Can you work these out from the model? Positions are in its coordinate system, mm. A direction names the side the tool comes from. Coordinates: 2 decimals unless noted, no trailing zeros. Order: outer loops, then holes, each group sorted by start corner. A loop starts at its lowest first (then second) coordinate and runs counter-clockwise, first axis right, second up. Notation, with made-up numbers: (86.25, 23) -> (140.25, 23) arc R13 ccw to (140.25, 48) -> close; hole circle Ø10 at (73, -7.5). An arc over 180 degrees is marked (long way). Write item = value, one per line. Start each with the question number.
Autodesk Inventor part; units mm, degrees
ref_plane "YZ Plane" through (0, 0, 0) normal (1, 0, 0) x (0, 1, 0)
ref_plane "XZ Plane" through (0, 0, 0) normal (0, 1, 0) x (-1, 0, 0)
ref_plane "XY Plane" through (0, 0, 0) normal (0, 0, 1) x (1, 0, 0)
sketch "Sketch1" plane through (0, 0, 0) normal (0, 0, 1) x (1, 0, 0)
  line L0 (-60.5, -49.5) -> (60.5, -49.5)
  line L1 (60.5, -49.5) -> (60.5, 49.5)
  line L2 (60.5, 49.5) -> (-60.5, 49.5)
  line L3 (-60.5, 49.5) -> (-60.5, -49.5)
  line L4 (-60.5, -49.5) -> (60.5, 49.5) construction
  line L5 (60.5, -49.5) -> (-60.5, 49.5) construction
  point P0 (0, 0)
  dimension "d0" = 121
  dimension "d1" = 99
extrude "Extrusion1" add sketch "Sketch1" along normal blind 37
sketch "Sketch3" plane through (0, 0, 37) normal (0, 0, 1) x (1, 0, 0)
  line L0 (-58.5, -47.5) -> (58.5, -47.5)
  line L1 (58.5, -47.5) -> (58.5, 47.5)
  line L2 (58.5, 47.5) -> (-58.5, 47.5)
  line L3 (-58.5, 47.5) -> (-58.5, -47.5)
  line L4 (-58.5, -47.5) -> (58.5, 47.5) construction
  line L5 (58.5, -47.5) -> (-58.5, 47.5) construction
  point P0 (0, 0)
  dimension "d8" = 117
  dimension "d9" = 95
extrude "Extrusion3" cut sketch "Sketch3" against normal blind 35.3
sketch "Sketch4" plane through (0, 0, 1.7) normal (0, 0, 1) x (1, 0, 0)
  line L0 (5.5, -22.5) -> (8.5, -22.5)
  line L1 (8.5, -22.5) -> (8.5, 22.5)
  line L2 (8.5, 22.5) -> (5.5, 22.5)
  line L3 (5.5, 22.5) -> (5.5, -22.5)
  line L4 (5.5, -22.5) -> (8.5, 22.5) construction
  line L5 (8.5, -22.5) -> (5.5, 22.5) construction
  line L6 (-58.5, -47.5) -> (-58.5, 47.5)
  point P0 (0, 0)
  point P1 (7, 0)
  dimension "d12" = 3
  dimension "d13" = 65.5
  dimension "d14" = 45
extrude "Extrusion4" add sketch "Sketch4" along normal blind 4
sketch "Sketch5" plane through (-60.5, 49.5, 0) normal (0, -1, 0) x (1, 0, 0)
  circle A0 centre (79, 8.7) radius 3
  line L0 (119, 1.7) -> (2, 1.7)
  line L1 (69, 1.7) -> (69, 5.7)
  point P0 (60.5, 0)
  dimension "d17" = 6
  dimension "d18" = 7
  dimension "d19" = 10
extrude "Extrusion5" cut sketch "Sketch5" along normal blind 4
sketch "Sketch6" plane through (-60.5, 49.5, 0) normal (0, -1, 0) x (1, 0, 0)
  line L0 (89.25, 5.5) -> (108.75, 5.5)
  line L1 (108.75, 5.5) -> (108.75, 18.5)
  line L2 (108.75, 18.5) -> (89.25, 18.5)
  line L3 (89.25, 18.5) -> (89.25, 5.5)
  line L4 (89.25, 5.5) -> (108.75, 18.5) construction
  line L5 (108.75, 5.5) -> (89.25, 18.5) construction
  line L6 (0, 0) -> (121, 0)
  circle A0 centre (79, 8.7) radius 3
  point P0 (60.5, 0)
  point P1 (99, 12)
  point P2 (79, 9)
  dimension "d23" = 19.5
  dimension "d24" = 13
  dimension "d25" = 12
  dimension "d26" = 20
extrude "Extrusion6" cut sketch "Sketch6" along normal blind 4 contours L3 L2 L1 L0
sketch "Sketch9" plane through (60.5, -49.5, 0) normal (1, 0, 0) x (0, 0, -1)
  line L0 (-25, 43.5) -> (-29, 43.5)
  line L1 (-29, 43.5) -> (-29, 55.5)
  line L2 (-29, 55.5) -> (-25, 55.5)
  line L3 (-25, 55.5) -> (-25, 43.5)
  line L4 (-25, 43.5) -> (-29, 55.5) construction
  line L5 (-29, 43.5) -> (-25, 55.5) construction
  line L6 (-37, 0) -> (-37, 99)
  point P0 (0, 49.5)
  point P1 (-27, 49.5)
  point P2 (-27, 49.5)
  point P3 (-37, 49.5)
  dimension "d37" = 12
  dimension "d38" = 4
  dimension "d39" = 10
extrude "Extrusion8" cut sketch "Sketch9" against normal blind 10
fillet "Fillet2" radius 2 4 edges at (-60.5, -49.5, 18.5) (60.5, -49.5, 18.5) (60.5, 49.5, 18.5) (-60.5, 49.5, 18.5)
sketch "Sketch10" plane through (0, 0, 1.7) normal (0, 0, 1) x (1, 0, 0)
  line L0 (-48.5, 37.5) -> (-4.5, 37.5)
  line L1 (-4.5, 37.5) -> (-4.5, -37.5)
  line L2 (-4.5, -37.5) -> (-48.5, -37.5)
  line L3 (-48.5, -37.5) -> (-48.5, 37.5)
  line L4 (-48.5, 37.5) -> (-4.5, -37.5) construction
  line L5 (-4.5, 37.5) -> (-48.5, -37.5) construction
  line L6 (5.5, 22.5) -> (5.5, -22.5)
  line L7 (-58.5, -47.5) -> (-58.5, 47.5)
  line L8 (58.5, -47.5) -> (-58.5, -47.5)
  line L9 (-58.5, 47.5) -> (58.5, 47.5)
  point P0 (0, 0)
  point P1 (-26.5, 0)
  dimension "d43" = 10
  dimension "d44" = 10
  dimension "d45" = 10
  dimension "d46" = 10
extrude "Extrusion9" cut sketch "Sketch10" against normal blind 10
sketch "Sketch12" plane through (-58.5, 49.5, 0) normal (0, 1, 0) x (1, 0, 0)
  line L0 (61, -28) -> (40, -28)
  line L1 (40, -28) -> (40, -8)
  line L2 (40, -8) -> (61, -8)
  line L3 (61, -8) -> (61, -28)
  line L4 (61, -28) -> (40, -8) construction
  line L5 (40, -28) -> (61, -8) construction
  line L6 (117, 0) -> (0, 0)
  point P0 (58.5, 0)
  point P1 (50.5, -18)
  point P2 (0, -37)
  dimension "d49" = 20
  dimension "d50" = 21
  dimension "d51" = 40
  dimension "d52" = 8
extrude "Extrusion10" cut sketch "Sketch12" against normal blind 10
fillet "Fillet3" radius 7 4 edges at (-4.5, 37.5, 0.85) (-48.5, 37.5, 0.85) (-48.5, -37.5, 0.85) (-4.5, -37.5, 0.85)
sketch "Sketch13" plane through (0, 0, 1.7) normal (0, 0, 1) x (1, 0, 0)
  line L0 (58.5, 47.5) -> (58.5, -47.5)
  line L1 (-58.5, 47.5) -> (58.5, 47.5)
  line L2 (58.5, -47.5) -> (-58.5, -47.5)
  line L3 (-58.5, -47.5) -> (-58.5, 47.5)
  point P0 (0, 0)
  point P1 (8.5, -42.5)
  point P2 (8.5, 42.5)
  point P3 (8.5, 22.5)
  point P4 (8.5, -22.5)
  dimension "d57" = 5
  dimension "d58" = 5
hole "Hole1" at (8.5, -42.5, 1.7) at (8.5, 42.5, 1.7) direction (0, 0, -1) diameter 4.496 end through all
equation "\"d65\" = Thickness"
equation "\"BendRadius\" = Thickness"
equation "\"BendReliefWidth\" = Thickness"
equation "\"BendReliefDepth\" = 0.5 * Thickness"
equation "\"CornerReliefSize\" = 4 * Thickness"
equation "\"MinimumRemnant\" = 2 * Thickness"
equation "\"TransitionRadius\" = BendRadius"
equation "\"JacobiRadiusSize\" = Thickness"
equation "\"GapSize\" = Thickness"
properties part number "_3DPrint"
(1) For P1, Ø1.6, axis at y = 48.5, z = 9, coming from the +X side; P2, Ø0.6, axis at y = 48, z = 10, coming from the -X side; P3, Ø8, axis at x = 17, y = 33, coming from the +Z side, each with a flat end and sliding along its axis, tell me the tip position at first contact or that it passes through.
(2) Thinking about a two-plate mould opening in X: for faces 1 (the face through (60.5, -1, 18)), 2 (the face through (-27, 48, 37)), 3 (the face through (-6.6, 35.5, 0.8)), 4 (the face through (-60.5, 1, 18)), which applies, +X half, -X half, draft (parallel to the pull), parting line (faces both ways), or undercut?
(3) Imagine slicing it at C-C (x = 4). Write out the boundary of the cut face in (y, z).
(4) Imagine slicing it at B-B (x = -20.5). Write out the boundary of the cut face in (y, z), plus the area to 3 significant figures.
(5) Imagine slicing it at A-A (y = 25). Write out the boundary of the cut face in (x, z).
(6) For faces 5 (the face through (-46.5, 35.4, 0.8)), 6 (the face through (7, 0, 5.7)), 7 (the face through (16.1, 48.5, 10.5)), which set-ups out of +Z, -Z, +X, -X, +Y, -Y let a thin tool reach every point of the face, with its end or its side?
(7) Imagine slicing it at D-D (y = -19). Write out the boundary of the cut face in (x, z).
(8) If I drill on L1, parallel to X at y = 6, z = 4; L2, parallel to X at y = 5.5, z = 11; L3, parallel to Y at x = -12, z = 35.5, over which ranges is the centre line in solid material (lowest first)? Write a range as from..to.
Result set:
q1.P1 = 60.49
q1.P2 = -60.49
q1.P3 = 1.7
q2.face_1 = +X half
q2.face_2 = draft
q2.face_3 = undercut
q2.face_4 = -X half
q3.outline = (-49.5, 0) -> (49.5, 0) -> (49.5, 37) -> (47.5, 37) -> (47.5, 1.7) -> (-47.5, 1.7) -> (-47.5, 37) -> (-49.5, 37) -> close
q4.outline = (-49.5, 0) -> (-37.5, 0) -> (-37.5, 1.7) -> (-47.5, 1.7) -> (-47.5, 37) -> (-49.5, 37) -> close; (37.5, 0) -> (49.5, 0) -> (49.5, 37) -> (47.5, 37) -> (47.5, 1.7) -> (37.5, 1.7) -> close
q4.area = 182 mm2
q5.outline = (-60.5, 0) -> (-48.5, 0) -> (-48.5, 1.7) -> (-58.5, 1.7) -> (-58.5, 37) -> (-60.5, 37) -> close; (-4.5, 0) -> (60.5, 0) -> (60.5, 37) -> (58.5, 37) -> (58.5, 1.7) -> (-4.5, 1.7) -> close
q6.face_5 = +Z, -Z
q6.face_6 = +Z
q6.face_7 = +Y
q7.outline = (-60.5, 0) -> (-48.5, 0) -> (-48.5, 1.7) -> (-58.5, 1.7) -> (-58.5, 37) -> (-60.5, 37) -> close; (-4.5, 0) -> (60.5, 0) -> (60.5, 37) -> (58.5, 37) -> (58.5, 1.7) -> (8.5, 1.7) -> (8.5, 5.7) -> (5.5, 5.7) -> (5.5, 1.7) -> (-4.5, 1.7) -> close
q8.L1 = -60.5..-58.5, 5.5..8.5, 58.5..60.5
q8.L2 = -60.5..-58.5, 58.5..60.5
q8.L3 = -49.5..-47.5, 47.5..49.5
